from build123d import *

# Parameters (mm, degrees)
BASE_FLANGE1_DEPTH           = 70
EDGE_FLANGE1_STRIP_W         = 9.4732
EDGE_FLANGE1_STRIP_H         = 2
EDGE_FLANGE1_STRIP_CUT_DEPTH = 132.921562236
EDGE_FLANGE1_DEPTH           = 132.921562236


# Sheet-metal steps are written as plain solids
with BuildPart() as part:
    # Sketch1 → Base-Flange1 (new body)
    with BuildSketch(Plane(origin=(0, 0, 0), x_dir=(1, 0, 0), z_dir=(0, 1, 0))):
        with BuildLine():
            Line((0, 77.222396617), (0, 0.7366))
            ThreePointArc((0, 0.7366), (0.215745145, 0.215745145), (0.7366, 0))
            Line((0.7366, 0), (133.658162236, 0))
            ThreePointArc((133.658162236, 0), (134.179017091, 0.215745145), (134.394762236, 0.7366))
            Line((134.394762236, 0.7366), (134.394762236, 77.222396617))
            Line((134.394762236, 77.222396617), (136.394762236, 77.222396617))
            Line((136.394762236, 77.222396617), (136.394762236, 0.7366))
            ThreePointArc((136.394762236, 0.7366), (135.593230653, -1.198468417), (133.658162236, -2))
            Line((133.658162236, -2), (0.7366, -2))
            ThreePointArc((0.7366, -2), (-1.198468417, -1.198468417), (-2, 0.7366))
            Line((-2, 0.7366), (-2, 77.222396617))
            Line((-2, 77.222396617), (0, 77.222396617))
        make_face()
    extrude(amount=BASE_FLANGE1_DEPTH)

    # Edge-Flange1 strip (across the edge) → Edge-Flange1 strip cut (cut)
    with BuildSketch(Plane(origin=(0.7366, 70, 0), x_dir=(0, -1, 0), z_dir=(1, 0, 0))):
        with Locations((-2, -1)):
            Rectangle(EDGE_FLANGE1_STRIP_W, EDGE_FLANGE1_STRIP_H)
    extrude(amount=EDGE_FLANGE1_STRIP_CUT_DEPTH, mode=Mode.SUBTRACT)

    # Edge-Flange1 section (across the edge) → Edge-Flange1 (add)
    with BuildSketch(Plane(origin=(0.7366, 70, 0), x_dir=(0, -1, 0), z_dir=(1, 0, 0))):
        with BuildLine():
            Line((0, 0.7366), (0, 28))
            Line((0, 28), (2, 28))
            Line((2, 28), (2, 0.7366))
            ThreePointArc((2, 0.7366), (2.215745145, 0.215745145), (2.7366, 0))
            Line((2.7366, 0), (2.7366, -2))
            ThreePointArc((2.7366, -2), (0.801531583, -1.198468417), (0, 0.7366))
        make_face()
    extrude(amount=EDGE_FLANGE1_DEPTH)


solid = part.part
Design review of the part built by this model. Coordinates are the model's own, in mm. A direction names the side the tool comes from. Coordinates: 2 decimals unless noted, no trailing zeros. Write each loop counter-clockwise with the first axis right and the second up, starting at its lowest first coordinate (ties: lowest second). Pieces come first, ordered by that corner, then holes. Notation, with made-up numbers: (72, -9.75) -> (107, -9.75) arc R22 ccw to (107, 12.25) -> close; hole circle Ø8 at (48.25, 26.25). An arc over 180 degrees is marked (long way). Write each question's results on one line, items separated by ' | '. Start each with the question number.
(1) Take a section at D-D on y = 6.5. Write out the cut boundary in (x, z).
(2) Take a section at B-B on x = 121.5. Write out the cut boundary in (y, z), and give its area (3 significant figures).
(3) Tool access review of faces 5 (the face through (0, 35, -40)), 6 (the face through (67.5, 0, 0.3)), 7 (the face through (66, 68, -15)): name each direction out of +Z, -Z, +X, -X, +Y, -Y from which nothing blocks a thin tool from reaching the whole face with its end or side.
(4) Clearance check with flat-ended pins moving along their axes: P1, Ø0.6, axis at y = 68.5, z = 1, coming from the -X side; P2, Ø3, axis at x = 72, z = -12, coming from the -Y side; P3, Ø2, axis at x = 44, y = 69, coming from the -Z side. State where each tip first meets the part, or that it passes through.
(5) The part is to be moulded in two halves that separate along X. For faces 1 (the face through (133.658, 69, -14)), 2 (the face through (66.267, 69.177, 1.22)), 3 (the face through (-2, 35, -38)), 4 (the face through (136.395, 35, -40)), say which applies: pulls with the +X half, pulls with the -X half, needs draft (parallel to the pull), parting line crosses it, or undercut.
(6) Take a section at A-A on z = -15.5. Write out the cut boundary in (x, y).
(7) For line 1 along X through (y, z) = (25, -25); line 2 along Z through (x, y) = (78, 61); line 3 along Y through (x, z) = (127, -11), list the stretches that pass through material, from the lowest coordinate up. Write a range as from..to.
(8) Take a section at C-C on z = -40.5. Write out the cut boundary in (x, y), and give its area (3 significant figures).
Results found:
1) outline: (-2, -77.22) -> (0, -77.22) -> (0, -0.74) arc R0.74 cw to (0.74, 0) -> (133.66, 0) arc R0.74 cw to (134.39, -0.74) -> (134.39, -77.22) -> (136.39, -77.22) -> (136.39, -0.74) arc R2.74 ccw to (133.66, 2) -> (0.74, 2) arc R2.74 ccw to (-2, -0.74) -> close
2) outline: (0, 0) -> (67.26, 0) arc R0.74 cw to (68, -0.74) -> (68, -28) -> (70, -28) -> (70, -0.74) arc R2.74 ccw to (67.26, 2) -> (0, 2) -> close | area: 195 mm2
3) face 5: -Z, +Y, -Y | face 6: +Z, -Z, +X, -X, -Y | face 7: -Z, -Y
4) P1: stops at x = -1.59 | P2: stops at y = 68 | P3: stops at z = -28
5) face 1: undercut | face 2: undercut | face 3: pulls with the -X half | face 4: pulls with the +X half
6) outline: (-2, 0) -> (0, 0) -> (0, 70) -> (-2, 70) -> close; (0.74, 68) -> (133.66, 68) -> (133.66, 70) -> (0.74, 70) -> close; (134.39, 0) -> (136.39, 0) -> (136.39, 70) -> (134.39, 70) -> close
7) line 1: x = -2..0, 134.39..136.39 | line 2: z = 0..2 | line 3: y = 68..70
8) outline: (-2, 0) -> (0, 0) -> (0, 70) -> (-2, 70) -> close; (134.39, 0) -> (136.39, 0) -> (136.39, 70) -> (134.39, 70) -> close | area: 280 mm2
